For this review, take the finished solid that the model builds, in its own axes (mm). Coordinates: 2 decimals unless noted, no trailing zeros. Loops run counter-clockwise (first coordinate to the right, second up) from the corner with the lowest first, then second, coordinate; pieces in that order, holes last. Notation, with made-up numbers: (57, -2) -> (93, -2) arc R21 cw to (93, 35) -> close; hole circle Ø6 at (-10, 18.5). An arc over 180 degrees is marked (long way). Use a Markdown table: item, result.
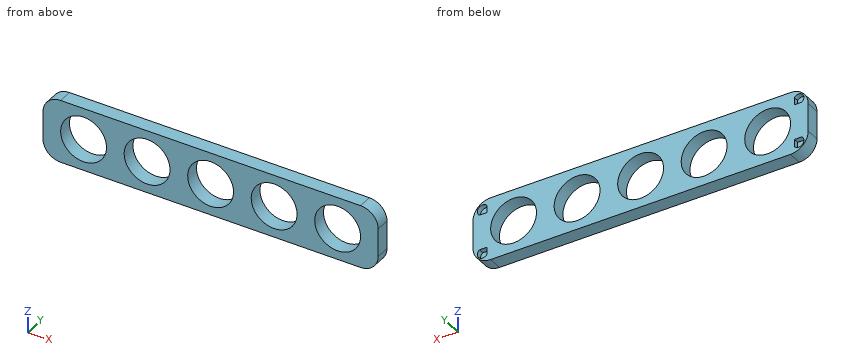
from build123d import *

# Parameters (mm, degrees)
SKETCH5_W           = 190
SKETCH5_H           = 36
BOSS_EXTRUDE1_DEPTH = 8
SKETCH6_R           = 13
SKETCH6_R_2         = 12.99768992
CUT_EXTRUDE1_DEPTH  = 8
FILLET2_R           = 10
CUT_EXTRUDE2_DEPTH  = 3


with BuildPart() as part:
    # Sketch5 → Boss-Extrude1 (new body)
    with BuildSketch(Plane(origin=(0, 0, 0), x_dir=(1, 0, 0), z_dir=(0, 1, 0))):
        with Locations((95, 18)):
            Rectangle(SKETCH5_W, SKETCH5_H)
    extrude(amount=BOSS_EXTRUDE1_DEPTH)

    # Sketch6 → Cut-Extrude1 (cut)
    with BuildSketch(Plane(origin=(0, 8, 0), x_dir=(1, 0, 0), z_dir=(0, 1, 0))):
        with Locations(Location((23, 18, 0), (0, 0, 270))):
            Circle(SKETCH6_R)
        with Locations(Location((59, 18, 0), (0, 0, 270))):
            Circle(SKETCH6_R)
        with Locations(Location((95.004620161, 18, 0), (0, 0, 270))):
            Circle(SKETCH6_R)
        with Locations(Location((131.004620161, 18, 0), (0, 0, 270))):
            Circle(SKETCH6_R)
        with Locations(Location((167.00231008, 18, 0), (0, 0, 270))):
            Circle(SKETCH6_R_2)
    extrude(amount=-CUT_EXTRUDE1_DEPTH, mode=Mode.SUBTRACT)

    # Fillet2
    fillet2_edges = [part.edges().sort_by_distance(p)[0] for p in [
        (0, 4, -36),
        (190, 4, -36),
        (190, 4, 0),
        (0, 4, 0),
    ]]
    fillet(fillet2_edges, radius=FILLET2_R)

    # Sketch7 → Cut-Extrude2 (cut)
    with BuildSketch(Plane(origin=(0, 8, 0), x_dir=(1, 0, 0), z_dir=(0, 1, 0))):
        with BuildLine():
            Line((3.652564445, 28.100196169), (7.852564445, 28.100196169))
            Line((7.852564445, 28.100196169), (7.852564445, 32.300196169))
            ThreePointArc((7.852564445, 32.300196169), (3.324368465, 32.628392149), (3.652564445, 28.100196169))
        make_face()
        with BuildLine():
            Line((3.652564445, 7.899803831), (7.852564445, 7.899803831))
            Line((7.852564445, 7.899803831), (7.852564445, 3.699803831))
            ThreePointArc((7.852564445, 3.699803831), (3.324368465, 3.371607851), (3.652564445, 7.899803831))
        make_face()
        with BuildLine():
            Line((186.347435555, 28.100196169), (182.147435555, 28.100196169))
            Line((182.147435555, 28.100196169), (182.147435555, 32.300196169))
            ThreePointArc((182.147435555, 32.300196169), (186.675631535, 32.628392149), (186.347435555, 28.100196169))
        make_face()
        with BuildLine():
            Line((182.147435555, 7.899803831), (182.147435555, 3.699803831))
            ThreePointArc((182.147435555, 3.699803831), (186.675631535, 3.371607851), (186.347435555, 7.899803831))
            Line((186.347435555, 7.899803831), (182.147435555, 7.899803831))
        make_face()
    extrude(amount=-CUT_EXTRUDE2_DEPTH, mode=Mode.SUBTRACT)


solid = part.part
(1) For line 1 along X through (y, z) = (4.25, -18); line 2 along X through (y, z) = (2.5, -14.5); line 3 along Z through (x, y) = (132, 6.25), list the stretches that pass through material, from the lowest coordinate up.
Found:
| item | result |
|---|---|
| line 1 | x = 0 to 10, 36 to 46, 72 to 82, 108 to 118, 144 to 154, 180 to 190 |
| line 2 | x = 0 to 10.48, 35.52 to 46.48, 71.52 to 82.48, 107.52 to 118.48, 143.52 to 154.48, 179.52 to 190 |
| line 3 | z = -36 to -30.96, -5.04 to 0 |
(2) Take a section at C-C on y = 6.25. State how many separate pieces and enclosed holes the cut face has, plus the area to 3 significant figures.
Found:
| item | result |
|---|---|
| separate pieces | 1 |
| enclosed holes | 9 |
| area | 4,000 mm^2 |
(3) Take a section at B-B on z = -18. Write out the cut boundary in (x, y).
Found:
| item | result |
|---|---|
| outline | (0, 0) -> (10, 0) -> (10, 8) -> (0, 8) -> close; (36, 0) -> (46, 0) -> (46, 8) -> (36, 8) -> close; (72, 0) -> (82, 0) -> (82, 8) -> (72, 8) -> close; (108, 0) -> (118, 0) -> (118, 8) -> (108, 8) -> close; (144, 0) -> (154, 0) -> (154, 8) -> (144, 8) -> close; (180, 0) -> (190, 0) -> (190, 8) -> (180, 8) -> close |
(4) Take a section at A-A on x = 23. Write out the cut boundary in (y, z), plus the area to 3 significant figures.
Found:
| item | result |
|---|---|
| outline | (0, -36) -> (8, -36) -> (8, -31) -> (0, -31) -> close; (0, -5) -> (8, -5) -> (8, 0) -> (0, 0) -> close |
| area | 80.0 mm^2 |
(5) For pin 1 Ø4.5 at (x, z) = (5.5, -4.5) entering from +Y; pin 2 Ø1.5 at (x, y) = (5, 6.5) entering from +Z; pin 3 Ø1.6 at (x, z) = (5.5, -30.5) entering from +Y; pin 4 Ø2.5 at (y, z) = (6, -30.5) entering from -X, all flat-tipped, find the tip position at first contact; note any pin that passes through.
Found:
| item | result |
|---|---|
| pin 1 | stops at y = 8 |
| pin 2 | stops at z = -0.95 |
| pin 3 | stops at y = 5 |
| pin 4 | stops at x = 0.54 |
(6) Take a section at D-D on x = 140. Write out the cut boundary in (y, z), plus the area to 3 significant figures.
Found:
| item | result |
|---|---|
| outline | (0, -36) -> (8, -36) -> (8, -27.39) -> (0, -27.39) -> close; (0, -8.61) -> (8, -8.61) -> (8, 0) -> (0, 0) -> close |
| area | 138 mm^2 |
